The figure shows three views and two pictorial views of one solid part (mm, origin at its lowest corner). Answer the questions. Coordinates: 2 decimals unless noted, no trailing zeros. Loops run counter-clockwise (first coordinate to the right, second up) from the corner with the lowest first, then second, coordinate; pieces in that order, holes last. Notation, with made-up numbers: (12.25, -30.75) -> (50.25, -30.75) arc R19 ccw to (50.25, -21.75) -> close; hole circle Ø1 at (-7.75, 13.5). An arc over 180 degrees is marked (long way). Answer in a Markdown table with one row per item.
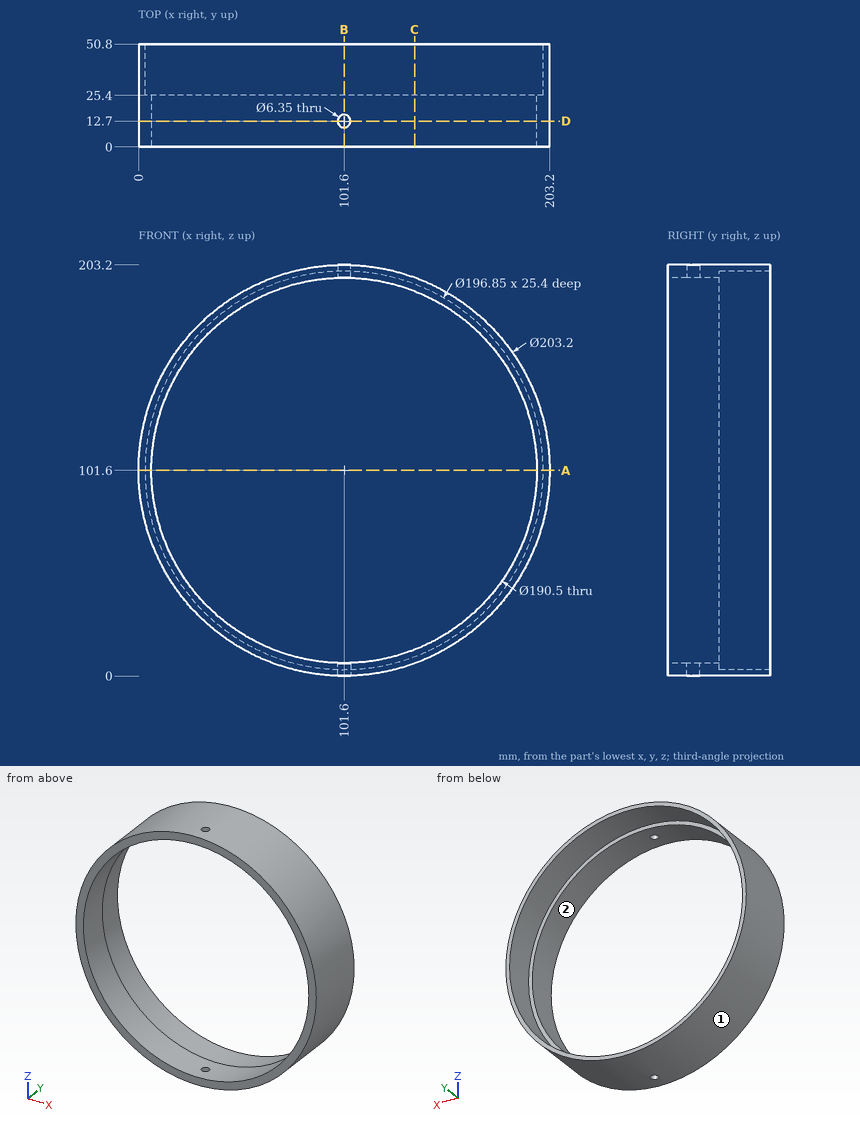
Item 1: A cutting plane is placed at C-C, the plane x = 136.5. Determine the outline of the cut face in (y, z), plus the area to 3 significant figures.
Findings below:
| item | result |
|---|---|
| outline | (0, 6.18) -> (50.8, 6.18) -> (50.8, 9.57) -> (25.4, 9.57) -> (25.4, 12.97) -> (0, 12.97) -> close; (0, 190.23) -> (25.4, 190.23) -> (25.4, 193.63) -> (50.8, 193.63) -> (50.8, 197.02) -> (0, 197.02) -> close |
| area | 517 mm2 |
Item 2: Flat-ended cylindrical pins translate along their axes: pin 1 Ø2 at (y, z) = (17.5, 52) entering from -X; pin 2 Ø2 at (y, z) = (22.5, 22.5) entering from -X; pin 3 Ø1.5 at (x, y) = (47, 23) entering from -Z; pin 4 Ø5 at (x, y) = (101.6, 12.7) entering from +Z. Find the tip coordinate at first contact, or state that the pin passes through.
Findings below:
| item | result |
|---|---|
| pin 1 | stops at x = 12.38 |
| pin 2 | stops at x = 36.62 |
| pin 3 | stops at z = 15.44 |
| pin 4 | passes through |
Item 3: Find the intervals of material crossed by probe 1 along Y at (x, z) = (101.6, 199.25) (3 decimals); probe 2 along Z at (x, y) = (101.6, 19.75); probe 3 along X at (y, z) = (41, 101), in increasing order.
Findings below:
| item | result |
|---|---|
| probe 1 | y = 0 to 9.525, 15.875 to 25.4 |
| probe 2 | z = 0 to 6.35, 196.85 to 203.2 |
| probe 3 | x = 0 to 3.18, 200.02 to 203.2 |
Item 4: A cutting plane is placed at D-D, the plane y = 12.7. Determine the outline of the cut face in (x, z) (3 decimals), plus the area to 3 significant figures.
Findings below:
| item | result |
|---|---|
| outline | (98.425, 0.05) -> (98.425, 6.403) arc R95.25 cw to (98.425, 196.797) -> (98.425, 203.15) arc R101.6 ccw to start; (104.775, 0.05) arc R101.6 ccw to (104.775, 203.15) -> (104.775, 196.797) arc R95.25 cw to (104.775, 6.403) -> close |
| area | 3,850 mm2 |
Item 5: Determine the mould class of the marked faces 1 and 2 for opening direction Z: +Z half, -Z half, draft (parallel to the pull), parting line (faces both ways), or undercut.
Findings below:
| item | result |
|---|---|
| face 1 | parting line |
| face 2 | undercut |
Item 6: A cutting plane is placed at B-B, the plane x = 101.6. Determine the outline of the cut face in (y, z) (3 decimals), plus the area to 3 significant figures.
Findings below:
| item | result |
|---|---|
| outline | (0, 0) -> (9.525, 0) -> (9.525, 6.35) -> (0, 6.35) -> close; (0, 196.85) -> (9.525, 196.85) -> (9.525, 203.2) -> (0, 203.2) -> close; (15.875, 0) -> (50.8, 0) -> (50.8, 3.175) -> (25.4, 3.175) -> (25.4, 6.35) -> (15.875, 6.35) -> close; (15.875, 196.85) -> (25.4, 196.85) -> (25.4, 200.025) -> (50.8, 200.025) -> (50.8, 203.2) -> (15.875, 203.2) -> close |
| area | 403 mm2 |
Item 7: A cutting plane is placed at A-A, the plane z = 101.6. Determine the outline of the cut face in (x, y) (3 decimals).
Findings below:
| item | result |
|---|---|
| outline | (0, 0) -> (6.35, 0) -> (6.35, 25.4) -> (3.175, 25.4) -> (3.175, 50.8) -> (0, 50.8) -> close; (196.85, 0) -> (203.2, 0) -> (203.2, 50.8) -> (200.025, 50.8) -> (200.025, 25.4) -> (196.85, 25.4) -> close |
